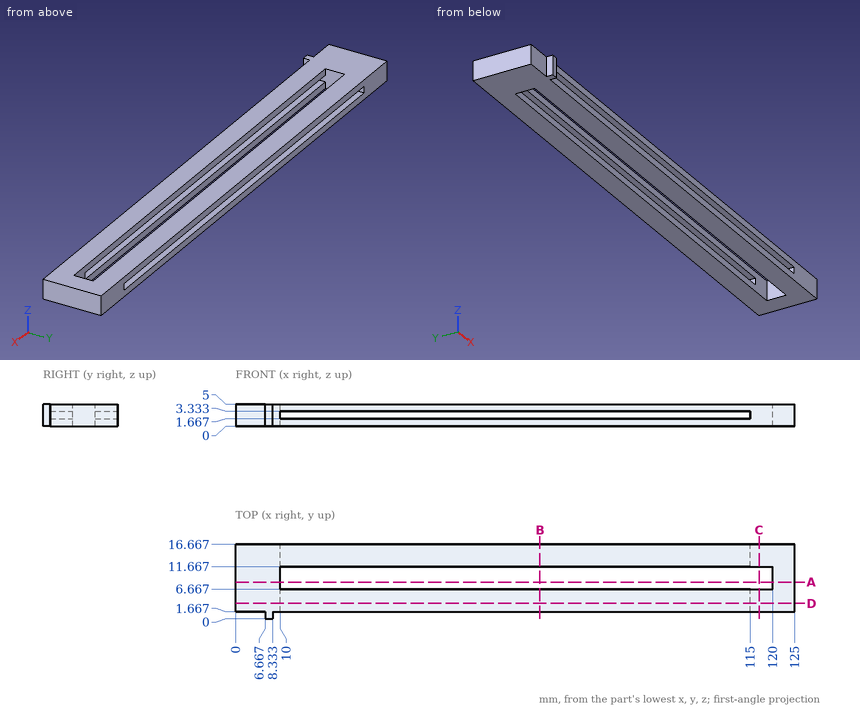
Design review of the part shown in the three views and the two pictorial views. Dimensions are in mm from the part's minimum x, y and z. Round coordinates to 2 decimals unless told otherwise and drop trailing zeros. Loops run counter-clockwise (first coordinate to the right, second up) from the corner with the lowest first, then second, coordinate; pieces in that order, holes last. Notation, with made-up numbers: M 14.5,-15 L 52.5,-15 A30 ccw 52.5,24 Z; hole C 41.25,81.25 d11. An arc over 180 degrees is marked long. Answer as a JSON object with one key per item and string values.
Item 1: We need section C-C, the plane x = 117. State the section outline as (y, z) points, and give its area (3 significant figures).
Check sheet entries:
{"outline": "M 1.67,0 L 6.67,0 L 6.67,5 L 1.67,5 Z; M 11.67,0 L 16.67,0 L 16.67,5 L 11.67,5 Z", "area": "50.0 mm2"}
Item 2: For line 1 along Z through (x, y) = (94, 3.25); line 2 along Y through (x, z) = (114, 3.4); line 3 along X through (y, z) = (10, 3.5), list the stretches that pass through material, from the lowest coordinate up.
Check sheet entries:
{"line 1": "0 to 1.67, 3.33 to 5", "line 2": "1.67 to 6.67, 11.67 to 16.67", "line 3": "0 to 10, 120 to 125"}
Item 3: We need section D-D, the plane y = 3.5. State the section outline as (x, z) points, and give its area (3 significant figures).
Check sheet entries:
{"outline": "M 0,0 L 125,0 L 125,5 L 0,5 Z; hole M 10,1.67 L 115,1.67 L 115,3.33 L 10,3.33 Z", "area": "450 mm2"}
Item 4: Clearance check with flat-ended pins moving along their axes: P1, Ø2.5, axis at x = 83.5, z = 2, coming from the -Y side; P2, Ø0.8, axis at y = 0.5, z = 2, coming from the +X side. State where each tip first meets the part, or that it passes through.
Check sheet entries:
{"P1": "y = 1.67", "P2": "x = 8.33"}
Item 5: We need section A-A, the plane y = 8.25. State the section outline as (x, z) points.
Check sheet entries:
{"outline": "M 0,0 L 10,0 L 10,5 L 0,5 Z; M 120,0 L 125,0 L 125,5 L 120,5 Z"}
Item 6: We need section B-B, the plane x = 68. State the section outline as (y, z) points.
Check sheet entries:
{"outline": "M 1.67,0 L 6.67,0 L 6.67,1.67 L 1.67,1.67 Z; M 1.67,3.33 L 6.67,3.33 L 6.67,5 L 1.67,5 Z; M 11.67,0 L 16.67,0 L 16.67,1.67 L 11.67,1.67 Z; M 11.67,3.33 L 16.67,3.33 L 16.67,5 L 11.67,5 Z"}
